```python
from build123d import *

# Parameters (mm, degrees)
F1_DEPTH = 2000
F3_DEPTH = 550
F5_DEPTH = 512.001


with BuildPart() as f1:
    # F0 (on Right) → F1 (new body)
    with BuildSketch(Plane.YZ):
        with BuildLine():
            ThreePointArc((0, 250), (250, 0), (0, -250))
            Line((0, -250), (-60, -250))
            Line((-60, -250), (-60, -256))
            Line((-60, -256), (0, -256))
            ThreePointArc((0, -256), (256, 0), (0, 256))
            Line((0, 256), (-60, 256))
            Line((-60, 256), (-60, 250))
            Line((-60, 250), (0, 250))
        make_face()
    extrude(amount=F1_DEPTH)

    # F2 (on face) → F3 (cut)
    with BuildSketch(Plane.XY.offset(256)):
        Polygon((0, 0), (60, 0), (316, 256), (0, 256), align=None)
        Polygon((0, 0), (0, -60), (60, 0), align=None)
    extrude(amount=-F3_DEPTH, mode=Mode.SUBTRACT)

    # F4 (on face) → F5 (cut, through all)
    with BuildSketch(Plane.XY.offset(256)):
        with BuildLine():
            Line((244, -12), (244, -60))
            Line((244, -60), (256, -60))
            Line((256, -60), (256, -12))
            ThreePointArc((256, -12), (250, -6), (244, -12))
        make_face()
        with BuildLine():
            Line((744, -12), (744, -60))
            Line((744, -60), (756, -60))
            Line((756, -60), (756, -12))
            ThreePointArc((756, -12), (750, -6), (744, -12))
        make_face()
        with BuildLine():
            Line((1244, -12), (1244, -60))
            Line((1244, -60), (1256, -60))
            Line((1256, -60), (1256, -12))
            ThreePointArc((1256, -12), (1250, -6), (1244, -12))
        make_face()
        with BuildLine():
            Line((1744, -60), (1756, -60))
            Line((1756, -60), (1756, -12))
            ThreePointArc((1756, -12), (1750, -6), (1744, -12))
            Line((1744, -12), (1744, -60))
        make_face()
    extrude(amount=-F5_DEPTH, mode=Mode.SUBTRACT)


solid = f1.part
```
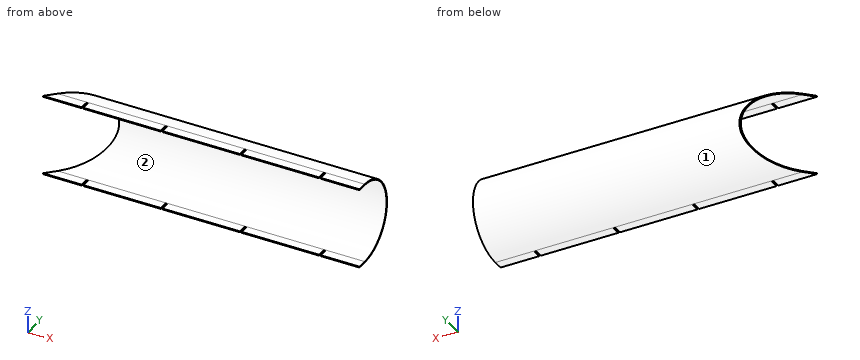
Input: part model. Units: mm. Frame: model coordinates. Face numbers are marked on the shaded views. Round coordinates to 2 decimals unless told otherwise and drop trailing zeros. Loops run counter-clockwise (first coordinate to the right, second up) from the corner with the lowest first, then second, coordinate; pieces in that order, holes last. Notation, with made-up numbers: (-1.75, 57) -> (40.25, 57) arc R25 ccw to (40.25, 88) -> close; hole circle Ø9 at (6.25, 43.5). An arc over 180 degrees is marked (long way). One line per item, written item: value.
(1) Section D-D (y = 173). Return the cut outline in (x, z), plus the area to 3 significant figures.
Geometry check:
outline: (233, -188.7) -> (2000, -188.7) -> (2000, -180.47) -> (233, -180.47) -> close; (233, 180.47) -> (2000, 180.47) -> (2000, 188.7) -> (233, 188.7) -> close
area: 29,100 mm2
(2) Pin query (flat end, axial travel): pin 1 (8 mm diameter, centred on x = 523.5, y = 153, fed in from +Z); pin 2 (4 mm diameter, centred on x = 430, z = 133, fed in from +Y); pin 3 (5 mm diameter, centred on y = -39, z = 252.5, fed in from -X). Return the tip coordinate at first contact, or that it passes through.
Geometry check:
pin 1: z = 208.17
pin 2: y = 219.94
pin 3: x = 18.5
(3) Section B-B (x = 815). Return the cut outline in (y, z), plus the area to 3 significant figures.
Geometry check:
outline: (-60, -256) -> (0, -256) arc R256 ccw to (0, 256) -> (-60, 256) -> (-60, 250) -> (0, 250) arc R250 cw to (0, -250) -> (-60, -250) -> close
area: 5,490 mm2
(4) Mould query, pull axis Z, two halves, no side actions, for the marked faces 1 and 2. Classes: pulls with the +Z half, pulls with the -Z half, needs draft (parallel to the pull), parting line crosses it, or undercut.
Geometry check:
face 1: parting line crosses it
face 2: undercut
(5) Section C-C (z = 0). Return the cut outline in (x, y), plus the area to 3 significant figures.
Geometry check:
outline: (310, 250) -> (2000, 250) -> (2000, 256) -> (316, 256) -> close
area: 10,100 mm2
(6) Section A-A (y = 36). Return the cut outline in (x, z).
Geometry check:
outline: (96, -253.46) -> (2000, -253.46) -> (2000, -247.39) -> (96, -247.39) -> close; (96, 247.39) -> (2000, 247.39) -> (2000, 253.46) -> (96, 253.46) -> close
(7) Material intervals for line 1 (Z direction, x = 1597, y = 8); line 2 (Z direction, x = 1033.5, y = 181); line 3 (Y direction, x = 1428, z = 22.5), sorted ascending. Write a range as [from, to].
Geometry check:
line 1: [-255.87, -249.87], [249.87, 255.87]
line 2: [-181.04, -172.45], [172.45, 181.04]
line 3: [248.99, 255.01]
